Verification items for the finished model (mm, model axes). Face numbers are marked on the shaded views. A direction names the side the tool comes from. Round coordinates to 2 decimals unless told otherwise and drop trailing zeros. Order: outer loops, then holes, each group sorted by start corner. A loop starts at its lowest first (then second) coordinate and runs counter-clockwise, first axis right, second up. Notation, with made-up numbers: (-33.5, 86.25) -> (-25.5, 86.25) arc R13 cw to (-25.5, 110.25) -> close; hole circle Ø7 at (-24, -2.5). An arc over 180 degrees is marked (long way). Return JSON: item names as keys, results as strings. Group by question number.
1) Draft check along Z on the marked faces 3, 4 and 5. Enter one of: pulls with the +Z half, pulls with the -Z half, needs draft (parallel to the pull), parting line crosses it, or undercut.
2) Tool access check on the marked faces 1 and 2. Record the directions out of +Z, -Z, +X, -X, +Y, -Y that give a thin tool (end or side, any length) a straight path to the whole face; none if there is none.
3) Section check B-B on x = -10. Enter the section's corners in (y, z) (3 decimals), plus the area to 3 significant figures.
4) Section check C-C on x = 14.5. Enter the section's corners in (y, z) (3 decimals).
5) Section check A-A on z = 0. Enter the section's corners in (x, y) (3 decimals), plus the area to 3 significant figures.
6) Scan lines: L1, parallel to Z at x = -10, y = -11.5 (3 decimals); L2, parallel to Z at x = 18, y = -6.5 (3 decimals); L3, parallel to Z at x = 4, y = -21. Record each from-to range of solid material in increasing order.
7) Depth check by flat-ended pin: pin 1 (4.5 mm diameter, centred on x = -4, z = -12, fed in from -Y); pin 2 (12 mm diameter, centred on y = -19, z = 8.5, fed in from +X); pin 3 (8 mm diameter, centred on x = 14, z = -11.5, fed in from -Y). Enter the tip coordinate at first touch or a pass-through.
8) Section check D-D on z = 19. Enter the section's corners in (x, y) (3 decimals).
```python
from build123d import *

# Parameters (mm, degrees)
BOSS_EXTRUDE2_DEPTH      = 25.4
BOSS_EXTRUDE2_DEPTH_BACK = 25.4
SKETCH3_R                = 3.175
CUT_EXTRUDE1_DEPTH       = 50.8
BOSS_EXTRUDE3_DEPTH      = 6.35
SKETCH4_R                = 6.35
CUT_EXTRUDE2_DEPTH       = 50.8
SKETCH8_R                = 3.175
CUT_EXTRUDE3_DEPTH       = 61.630559774


with BuildPart() as part:
    # Sketch1 → Boss-Extrude2 (new, two sides: drawn at the far end of the back side and taken through both)
    with BuildSketch(Plane(origin=(0, 0, 0), x_dir=(0, 0, -1), z_dir=(1, 0, 0)).offset(-BOSS_EXTRUDE2_DEPTH_BACK)):
        Polygon((18.17497, -22.225), (24.52497, -22.225), (24.52497, 0), (-24.52497, 0), (-24.52497, -22.225), (-18.17497, -22.225), (-18.17497, -6.35), (18.17497, -6.35), align=None)
    extrude(amount=BOSS_EXTRUDE2_DEPTH + BOSS_EXTRUDE2_DEPTH_BACK)

    # Sketch3 → Cut-Extrude1 (cut)
    with BuildSketch(Plane.XY.offset(24.52497)):
        with Locations((-15.875, -12.7)):
            Circle(SKETCH3_R)
        with Locations((15.875, -12.7)):
            Circle(SKETCH3_R)
    extrude(amount=-CUT_EXTRUDE1_DEPTH, mode=Mode.SUBTRACT)

    # Sketch7 → Boss-Extrude3 (add)
    with BuildSketch(Plane.XZ.offset(6.35)):
        Polygon((-25.4, 9.525), (0, 9.525), (25.4, 9.525), (25.4, -9.525), (-1.632648861, -9.525), (-25.4, -9.525), align=None)
    extrude(amount=BOSS_EXTRUDE3_DEPTH)

    # Sketch4 → Cut-Extrude2 (cut)
    with BuildSketch(Plane(origin=(0, 0, 0), x_dir=(1, 0, 0), z_dir=(0, 1, 0))):
        with Locations(Location((0, 0, 0), (0, 0, 270))):
            Circle(SKETCH4_R)
    extrude(amount=-CUT_EXTRUDE2_DEPTH, mode=Mode.SUBTRACT)

    # Sketch8 → Cut-Extrude3 (cut, through all)
    with BuildSketch(Plane.ZY.offset(25.4)):
        with Locations((0, -6.35)):
            Circle(SKETCH8_R)
    extrude(amount=-CUT_EXTRUDE3_DEPTH, mode=Mode.SUBTRACT)


solid = part.part
```
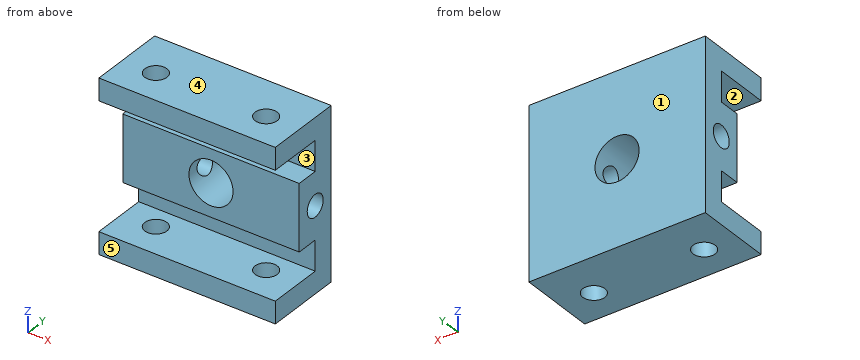
Check result:
{
 "1": {"face 3": "undercut", "face 4": "pulls with the +Z half", "face 5": "needs draft"},
 "2": {"face 1": "+Z, -Z, +X, -X, +Y", "face 2": "+X, -X, -Y"},
 "3": {"outline": "(-22.225, -24.525) -> (0, -24.525) -> (0, 24.525) -> (-22.225, 24.525) -> (-22.225, 18.175) -> (-6.35, 18.175) -> (-6.35, 9.525) -> (-12.7, 9.525) -> (-12.7, -9.525) -> (-6.35, -9.525) -> (-6.35, -18.175) -> (-22.225, -18.175) -> close; hole circle Ø6.35 at (-6.35, 0)", "area": "602 mm^2"},
 "4": {"outline": "(-22.225, -24.525) -> (-15.562, -24.525) -> (-15.562, -18.175) -> (-22.225, -18.175) -> close; (-22.225, 18.175) -> (-15.562, 18.175) -> (-15.562, 24.525) -> (-22.225, 24.525) -> close; (-12.7, -9.525) -> (-6.35, -9.525) -> (-6.35, -18.175) -> (-9.838, -18.175) -> (-9.838, -24.525) -> (0, -24.525) -> (0, 24.525) -> (-9.838, 24.525) -> (-9.838, 18.175) -> (-6.35, 18.175) -> (-6.35, 9.525) -> (-12.7, 9.525) -> close; hole circle Ø6.35 at (-6.35, 0)"},
 "5": {"outline": "(-25.4, -12.7) -> (-6.35, -12.7) -> (-6.35, -9.525) -> (-25.4, -9.525) -> close; (-25.4, -3.175) -> (-6.35, -3.175) -> (-6.35, 0) -> (-25.4, 0) -> close; (6.35, -12.7) -> (25.4, -12.7) -> (25.4, -9.525) -> (6.35, -9.525) -> close; (6.35, -3.175) -> (25.4, -3.175) -> (25.4, 0) -> (6.35, 0) -> close", "area": "242 mm^2"},
 "6": {"L1": "-24.525 to -18.175, -9.525 to 9.525, 18.175 to 24.525", "L2": "-24.525 to -18.175, -9.525 to -3.171, 3.171 to 9.525, 18.175 to 24.525", "L3": "-24.52 to -18.17, 18.17 to 24.52"},
 "7": {"pin 1": "y = -6.35", "pin 2": "through", "pin 3": "y = -12.7"},
 "8": {"outline": "(-25.4, -22.225) -> (25.4, -22.225) -> (25.4, 0) -> (-25.4, 0) -> close; hole circle Ø6.35 at (-15.875, -12.7); hole circle Ø6.35 at (15.875, -12.7)"}
}
